Part print with two shaded views. Sizes in mm from the minimum x, y, z corner. Round coordinates to 2 decimals unless told otherwise and drop trailing zeros. Order: outer loops, then holes, each group sorted by start corner. A loop starts at its lowest first (then second) coordinate and runs counter-clockwise, first axis right, second up. Notation, with made-up numbers: (61, 3) - (109, 3) arc R22 cw to (109, 15) - close; hole circle Ø10 at (-27.75, -36). An arc over 180 degrees is marked (long way). Use one line per item in the form item = value.
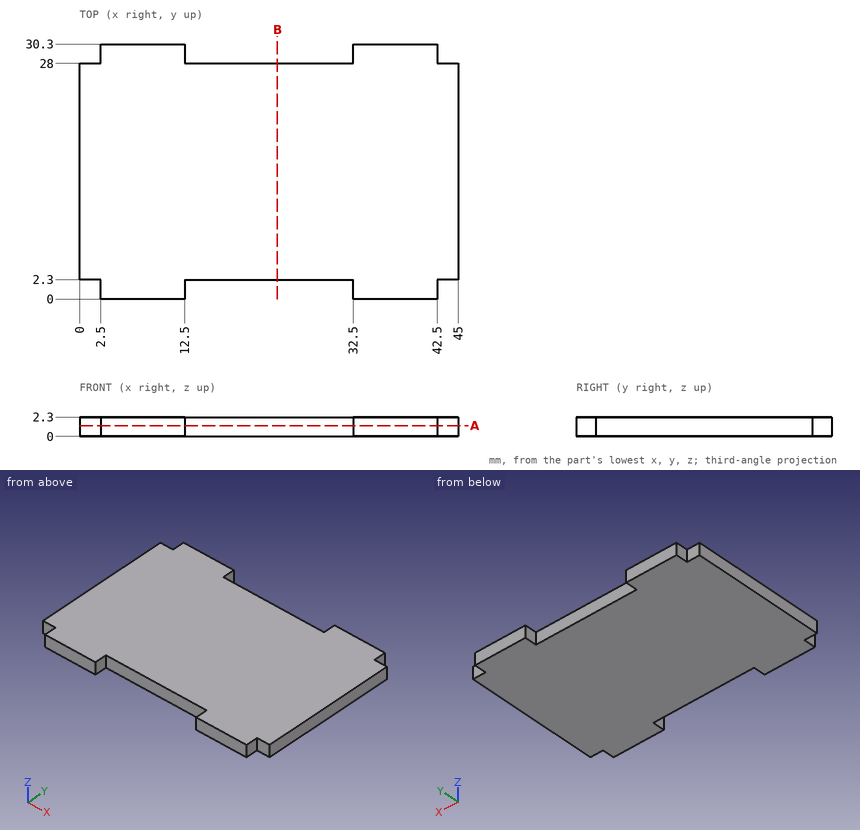
(1) Probe probe 1 along X at (y, z) = (2, 0.35); probe 2 along Y at (x, z) = (28, 2). List the from-to ranges inside material, lowest first. Write a range as [from, to].
Report:
probe_1 = [2.5, 12.5], [32.5, 42.5]
probe_2 = [2.3, 28]
(2) Slice it at B-B on x = 23.5. Give the cut face in (y, z).
Report:
outline = (2.3, 0) - (28, 0) - (28, 2.3) - (2.3, 2.3) - close
(3) Slice it at A-A on z = 1.3. Give the cut face in (x, y), then the cut area to 3 significant figures.
Report:
outline = (0, 2.3) - (2.5, 2.3) - (2.5, 0) - (12.5, 0) - (12.5, 2.3) - (32.5, 2.3) - (32.5, 0) - (42.5, 0) - (42.5, 2.3) - (45, 2.3) - (45, 28) - (42.5, 28) - (42.5, 30.3) - (32.5, 30.3) - (32.5, 28) - (12.5, 28) - (12.5, 30.3) - (2.5, 30.3) - (2.5, 28) - (0, 28) - close
area = 1,250 mm2
(4) Pin check, flat tips, straight feed: pin 1 (1.2 mm diameter, centred on y = 1.5, z = 1.5, fed in from -X); pin 2 (1.2 mm diameter, centred on x = 43.5, z = 1.5, fed in from -Y); pin 3 (1.2 mm diameter, centred on y = 1, z = 1.5, fed in from +X). Stop position of each tip, or through.
Report:
pin_1 = 2.5
pin_2 = 2.3
pin_3 = 42.5
